Model file for the job. Use its own axes, mm. A direction names the side the tool comes from. Coordinates: 2 decimals unless noted, no trailing zeros. Order: outer loops, then holes, each group sorted by start corner. A loop starts at its lowest first (then second) coordinate and runs counter-clockwise, first axis right, second up. Notation, with made-up numbers: (79.25, 62.5) -> (88.25, 62.5) arc R26 ccw to (88.25, 97.5) -> close; hole circle Ø4 at (42, -36.5). An arc over 180 degrees is marked (long way). Return JSON: item names as keys, results as strings. Group by question number.
1) Cut at B-B (z = -14.5). Write the cut outline in (x, y).
2) Cut at A-A (x = 100). Write the cut outline in (y, z).
3) Pull direction Y, two halves, no side cores. Call faces 4 (the flat face through (-2, 0, 0)), 5 (the flat face through (-135, -45, 0)), 6 (the flat face through (-150, -2, 0)): +Y half, -Y half, draft (parallel to the pull), parting line (faces both ways), or undercut.
4) Flat gauge pins, fed straight in: pin 1 (2 mm diameter, centred on x = 44, z = 0.5, fed in from +Y); pin 2 (13 mm diameter, centred on x = -100, z = 0, fed in from -Y); pin 3 (3 mm diameter, centred on y = -38.5, z = 11, fed in from -X); pin 4 (2 mm diameter, centred on y = -14.5, z = 5, fed in from +X). Where does each tip first touch, or does it go through?
5) Probe line 1 (Z direction, x = 100, y = -15); line 2 (X direction, y = -31, z = 6); line 3 (X direction, y = -13.5, z = -5). List the from-to ranges inside material, lowest first.
6) Which spindle directions (+Z, -Z, +X, -X, +Y, -Y) get a long thin tool onto all of the face, cutting with end or side? Do faces 1 (the cylindrical face through (89, -25, 0)), 2 (the flat face through (135, -5, 0)), 3 (the flat face through (-135, -5, 0)). Say none if no direction does.
7) Cut at C-C (y = -36.5). Write the cut outline in (x, z), and give its area (3 significant figures).
from build123d import *

# Parameters (mm, degrees)
F0_W     = 300
F0_H     = 45
F0_R     = 11
F1_DEPTH = 50
F2_W     = 40
F2_H     = 2.5
F2_H_2   = 45
F3_DEPTH = 30
F4_W     = 40
F4_H     = 45
F5_DEPTH = 30


with BuildPart() as f1:
    # F0 (on Front) → F1 (new body)
    with BuildSketch(Plane.XZ):
        Rectangle(F0_W, F0_H)
        with Locations((-100, 0)):
            Circle(F0_R, mode=Mode.SUBTRACT)
        with Locations((100, 0)):
            Circle(F0_R, mode=Mode.SUBTRACT)
    extrude(amount=F1_DEPTH)

    # F2 (on face) → F3 (cut)
    with BuildSketch(Plane(origin=(-150, 0, 0), x_dir=(0, -1, 0), z_dir=(-1, 0, 0))):
        with Locations((25, -23.75)):
            Rectangle(F2_W, F2_H)
        with Locations((25, 23.75)):
            Rectangle(F2_W, F2_H)
        with Locations((25, 0)):
            Rectangle(F2_W, F2_H_2)
    extrude(amount=-F3_DEPTH, mode=Mode.SUBTRACT)

    # F4 (on face) → F5 (cut)
    with BuildSketch(Plane.YZ.offset(150)):
        with Locations((-25, 0)):
            Rectangle(F4_W, F4_H)
    extrude(amount=-F5_DEPTH, mode=Mode.SUBTRACT)


solid = f1.part
Answers below:
{
 "1": {"outline": "(-150, -50) -> (150, -50) -> (150, -45) -> (120, -45) -> (120, -5) -> (150, -5) -> (150, 0) -> (-150, 0) -> (-150, -5) -> (-120, -5) -> (-120, -45) -> (-150, -45) -> close"},
 "2": {"outline": "(-50, -22.5) -> (0, -22.5) -> (0, -11) -> (-50, -11) -> close; (-50, 11) -> (0, 11) -> (0, 22.5) -> (-50, 22.5) -> close"},
 "3": {"face 4": "+Y half", "face 5": "undercut", "face 6": "draft"},
 "4": {"pin 1": "stops at y = 0", "pin 2": "passes through", "pin 3": "stops at x = -120", "pin 4": "stops at x = 120"},
 "5": {"line 1": "z = -22.5 to -11, 11 to 22.5", "line 2": "x = -120 to -109.22, -90.78 to 90.78, 109.22 to 120", "line 3": "x = -120 to -109.8, -90.2 to 90.2, 109.8 to 120"},
 "6": {"face 1": "+Y, -Y", "face 2": "+Z, -Z, +X", "face 3": "+Z, -Z, -X"},
 "7": {"outline": "(-120, -22.5) -> (120, -22.5) -> (120, 22.5) -> (-120, 22.5) -> close; hole circle Ø22 at (-100, 0); hole circle Ø22 at (100, 0)", "area": "10,000 mm^2"}
}
